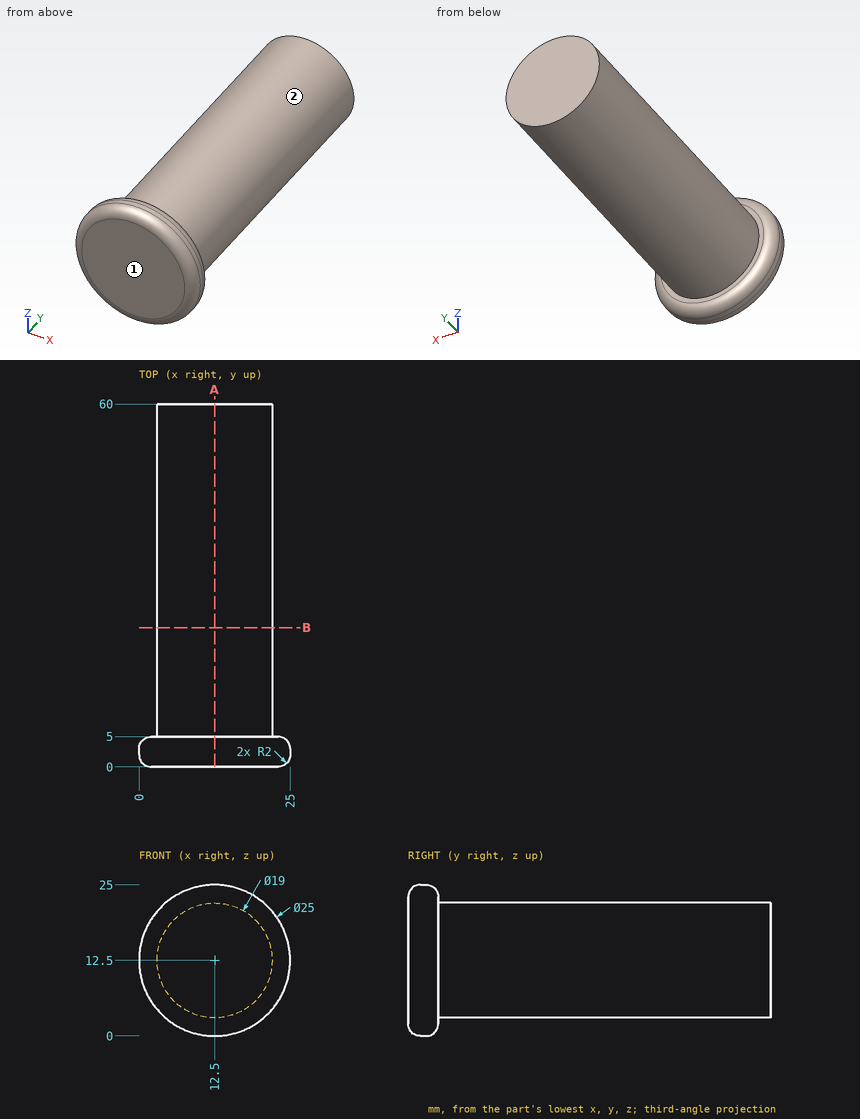
Drawing for the job (mm, zero at the part's lowest x, y, z). A direction names the side the tool comes from. Round coordinates to 2 decimals unless told otherwise and drop trailing zeros. Order: outer loops, then holes, each group sorted by start corner. A loop starts at its lowest first (then second) coordinate and runs counter-clockwise, first axis right, second up. Notation, with made-up numbers: (47, 48) -> (106, 48) arc R21 ccw to (106, 57) -> close; hole circle Ø9 at (16, 17.5). An arc over 180 degrees is marked (long way). Put each result on its own line as item: value.
Q1. Band-saw the part on A-A (x = 12.5). Give the cut face in (y, z), and give its area (3 significant figures).
From the geometry:
outline: (0, 2) arc R2 ccw to (2, 0) -> (3, 0) arc R2 ccw to (5, 2) -> (5, 3) -> (60, 3) -> (60, 22) -> (5, 22) -> (5, 23) arc R2 ccw to (3, 25) -> (2, 25) arc R2 ccw to (0, 23) -> close
area: 1,170 mm2
Q2. Band-saw the part on B-B (y = 23). Give the cut face in (x, z), and give its area (3 significant figures).
From the geometry:
outline: circle Ø19 at (12.5, 12.5)
area: 284 mm2
Q3. Wall check: line 1 (Y direction, x = 7.75, z = 21.25); line 2 (X direction, y = 30, z = 14); line 3 (Z direction, x = 5.75, y = 20). Give the ranges that are in metal, low to high. Write a range as [from, to].
From the geometry:
line 1: y = [0, 5]
line 2: x = [3.12, 21.88]
line 3: z = [5.82, 19.18]
Q4. Pin check, flat tips, straight feed: pin 1 Ø1.5 at (x, y) = (18.5, 27.5) entering from -Z; pin 2 Ø5 at (y, z) = (47, 17) entering from +X; pin 3 Ø5 at (x, y) = (8, 18.5) entering from +Z; pin 4 Ø1 at (x, z) = (18, 11) entering from -Y. Stop position of each tip, or through.
From the geometry:
pin 1: stops at z = 4.58
pin 2: stops at x = 21.79
pin 3: stops at z = 21.79
pin 4: stops at y = 0
Q5. Tool access for the marked faces 1 and 2: list every direction of +Z, -Z, +X, -X, +Y, -Y with a clear straight run to the whole face (end or side of a thin tool).
From the geometry:
face 1: +Z, -Z, +X, -X, -Y
face 2: +Y
